Read the model definition and answer for the solid it produces. Units are mm, in the model's axes. Round coordinates to 2 decimals unless told otherwise and drop trailing zeros. Order: outer loops, then holes, each group sorted by start corner. A loop starts at its lowest first (then second) coordinate and runs counter-clockwise, first axis right, second up. Notation, with made-up numbers: (9.5, 35) -> (66.5, 35) arc R21 cw to (66.5, 50) -> close; hole circle Ø8 at (-29.75, 56). An arc over 180 degrees is marked (long way). Use a Markdown table: item, result. Add a question column.
1. The mould has two halves that part along X. Classify faces 1 (the face through (4, 405.009, -1)), 2 (the face through (0.84, 199.67, 3.78)), 3 (the face through (3.51, 199.67, -3.22)): +X half, -X half, draft (parallel to the pull), parting line (faces both ways), or undercut.
2. Section B-B, the plane x = 0 is taken. Give the vertices of the cut face in (y, z), then the cut area to 3 significant figures.
3. Section C-C, the plane y = 291.5 is taken. Give the vertices of the cut face in (x, z) (1 decimal).
4. Section A-A, the plane z = 0 is taken. Give the vertices of the cut face in (x, y), then the cut area to 3 significant figures.
5. Consider L1, parallel to Z at x = -0.75, y = 174.5; L2, parallel to Z at x = 0.25, y = 67.5. Determine where each line is inside the solid, lowest interval first. Write a range as [from, to].
6. Given pin 1 (3 mm diameter, centred on y = 341, z = 2, fed in from -X); pin 2 (2 mm diameter, centred on x = 3.5, z = 0.5, fed in from +Y); pin 3 (5 mm diameter, centred on x = -3, y = 45, fed in from +Z); pin 4 (2 mm diameter, centred on x = -3, y = 334.5, fed in from +Z), each flat-ended and moving along its own axis, determine where each tip first touches the part or whether it passes through.
```python
from build123d import *

# Parameters (mm, degrees)
F0_R     = 4.7625
F0_R_2   = 3.8735
F1_DEPTH = 405.008555
F2_ANGLE = 30
F3_ANGLE = 30


with BuildPart() as f1:
    # F0 (on Front) → F1 (new body)
    with BuildSketch(Plane.XZ):
        Circle(F0_R)
        Circle(F0_R_2, mode=Mode.SUBTRACT)
    extrude(amount=-F1_DEPTH)


with BuildPart() as f1_1:
    # F2: moved
    add(f1.part.rotate(Axis((0, 0, 0), (0, -1, 0)), F2_ANGLE))


with BuildPart() as f1_2:
    # F3: moved
    add(f1_1.part.rotate(Axis((0, 0, 0), (0, -1, 0)), F3_ANGLE))


solid = f1_2.part
```
Verdict:
| question | item | result |
|---|---|---|
| 1 | face 1 | draft |
| 1 | face 2 | undercut |
| 1 | face 3 | parting line |
| 2 | outline | (0, -4.76) -> (405.01, -4.76) -> (405.01, -3.87) -> (0, -3.87) -> close; (0, 3.87) -> (405.01, 3.87) -> (405.01, 4.76) -> (0, 4.76) -> close |
| 2 | area | 720 mm2 |
| 3 | outline | circle Ø9.5 at (0, 0); hole circle Ø7.7 at (0, 0) |
| 4 | outline | (-4.76, 0) -> (-3.87, 0) -> (-3.87, 405.01) -> (-4.76, 405.01) -> close; (3.87, 0) -> (4.76, 0) -> (4.76, 405.01) -> (3.87, 405.01) -> close |
| 4 | area | 720 mm2 |
| 5 | L1 | z = [-4.7, -3.8], [3.8, 4.7] |
| 5 | L2 | z = [-4.76, -3.87], [3.87, 4.76] |
| 6 | pin 1 | stops at x = -4.74 |
| 6 | pin 2 | stops at y = 405.01 |
| 6 | pin 3 | stops at z = 4.74 |
| 6 | pin 4 | stops at z = 4.32 |
